Read the model definition and answer for the solid it produces. Units are mm, in the model's axes. A direction names the side the tool comes from. Coordinates: 2 decimals unless noted, no trailing zeros. Loops run counter-clockwise (first coordinate to the right, second up) from the corner with the lowest first, then second, coordinate; pieces in that order, holes last. Notation, with made-up numbers: (-36, 21.25) - (-29, 21.25) arc R26 ccw to (-29, 51.25) - close; hole circle Ø11 at (5, 65). An arc over 180 degrees is marked (long way). Use CSV: the item, a comma, the result in double quotes.
Autodesk Fusion 360 part; units mm, degrees
sketch "Sketch1" plane through (0, 0, 0) normal (0, 0, 1) x (1, 0, 0)
  circle A0 centre (0, 0) radius 5.95
  circle A1 centre (0, 0) radius 9
  circle A2 centre (0, 0) radius 10.35
  circle A3 centre (0, 0) radius 2.5
  circle A4 centre (0, 0) radius 3
  dimension "d1" = 11.9
  dimension "d2" = 18
  dimension "d3" = 20.7
  dimension "d8" = 5
  dimension "d9" = 6
extrude "Extrude1" add sketch "Sketch1" along normal blind 30 contours A0 | A2 | A4 makes body 1 at (10.2986, -1.0305, 20) makes body 2 at (5.9204, -0.5924, 20)
extrude "Extrude2" add sketch "Sketch1" along normal blind 28 contours A1 bodies 1 2
extrude "Extrude3" cut sketch "Sketch1" along normal blind 25 contours A3 | A4 bodies 1
chamfer "Chamfer1" distance 1 distance2 10 1 edges at (-9.6496, -3.7427, 30) measured on face at (9.828, -0.9613, 30) on bodies 1
sketch "Sketch2" plane through (0, 0, 0) normal (1, 0, 0) x (0, 0, -1)
  arc A0 (-38, -10) -> (-28, 0) centre (-38, 0) ccw
  line L0 (-28, 0) -> (-38, 0)
  line L1 (-38, 0) -> (-38, -10)
  line L2 (-1.75, 0) -> (-22.5, 0)
  line L3 (-28, 0) -> (-28, -12) construction
  circle A1 centre (-29.55, -7.342) radius 1.55
  dimension "d14" = 10
  dimension "d15" = 38
  dimension "d19" = 3.1
revolve "Revolve1" cut sketch "Sketch2" angle 360 about axis through (0, 0, 28) along (0, 0, 1) contours A0 L0 L1 A1 | A0 A1 picked at (-30.5667, -6.5077) bodies 1
equation "d1 = d2 - ( 2 * 3.05 ) * 1 mm"
equation "d8 = draadstang - 2 * draadstangtolerance"
equation "d9 = draadstang"
equation "draadstang = 6 mm"
equation "draadstangtolerance = 0.5 mm"
Q1. The part is cut by section C-C on z = 26. Determine the outline of the cut face in (x, y), and give its area (3 significant figures).
Reported:
outline,"circle Ø19.5 at (0, 0); hole circle Ø5 at (0, 0)"
area,"279 mm²"
Q2. The part is cut by section A-A on x = 0. Determine the outline of the cut face in (y, z), and give its area (3 significant figures).
Reported:
outline,"(-10.35, 0) - (-3, 0) - (-3, 25) - (-2.5, 25) - (-2.5, 28.32) arc R10 cw to (-5.95, 29.96) - (-5.95, 28) - (-9, 28) - (-9, 30) - (-9.35, 30) - (-10.35, 20) - close; (2.5, 25) - (3, 25) - (3, 0) - (10.35, 0) - (10.35, 20) - (9.35, 30) - (9, 30) - (9, 28) - (5.95, 28) - (5.95, 29.96) arc R10 cw to (2.5, 28.32) - close"
area,"417 mm²"
Q3. The part is cut by section D-D on z = 8. Determine the outline of the cut face in (x, y).
Reported:
outline,"circle Ø20.7 at (0, 0); hole circle Ø6 at (0, 0)"
Q4. Given P1, Ø1.5, axis at x = 5.5, z = 23.5, coming from the +Y side; P2, Ø2, axis at y = -2.5, z = 16, coming from the +X side; P3, Ø9, axis at x = 0, y = -0.5, coming from the +Z side, each flat-ended and moving along its own axis, determine where each tip first touches the part or whether it passes through.
Reported:
P1,"stops at y = 8.81"
P2,"stops at x = 10.24"
P3,"stops at z = 29.34"
Q5. Find the intervals of material crossed by probe 1 along Z at (x, y) = (3.75, 6.25); probe 2 along Y at (x, z) = (2, 13.25); probe 3 along Y at (x, z) = (0, 7), in increasing order. Write a range as [from, to].
Reported:
probe 1,"z = [0, 28]"
probe 2,"y = [-10.15, -2.24], [2.24, 10.15]"
probe 3,"y = [-10.35, -3], [3, 10.35]"
Q6. A tool of negligible diameter and unlimited length cuts with its end or side. For faces 1 (the face through (-8.21, 6.3, 9.86)), 2 (the face through (-3, 0, 12)), 3 (the face through (2, -6, 28)), from which of +Z, -Z, +X, -X, +Y, -Y can it reach the whole face along a straight path? Write none if from no direction.
Reported:
face 1,"+Z, -Z"
face 2,"-Z"
face 3,"+Z"
